Could you check a few things on this model? Use its own coordinates, in mm. Give positions to 0.01 mm unless a question says otherwise; leave off trailing zeros. Write each loop counter-clockwise with the first axis right and the second up, starting at its lowest first coordinate (ties: lowest second). Pieces come first, ordered by that corner, then holes. Notation, with made-up numbers: (-30.5, 7.25) - (17.5, 7.25) arc R36 ccw to (17.5, 45.25) - close; hole circle Ø5 at (39, 48). An arc over 180 degrees is marked (long way). Answer in a Markdown table with one row per item.
from build123d import *

# Parameters (mm, degrees)
F0_W     = 19
F0_H     = 35
F1_DEPTH = 6
F2_R     = 4
F3_R     = 3


with BuildPart() as f1:
    # F0 (on Front) → F1 (new body)
    with BuildSketch(Plane.XZ):
        with Locations((-4.541362, 17.316902)):
            Rectangle(F0_W, F0_H)
    extrude(amount=F1_DEPTH)

    # F2
    f2_edges = [f1.edges().sort_by_distance(p)[0] for p in [
        (4.958638, -3, 34.816902),
        (4.958638, -3, -0.183098),
        (-14.041362, -3, 34.816902),
        (-14.041362, -3, -0.183098),
    ]]
    fillet(f2_edges, radius=F2_R)

    # F3
    f3_edges = [f1.edges().sort_by_distance(p)[0] for p in [
        (-14.041362, -6, 17.316902),
    ]]
    fillet(f3_edges, radius=F3_R)


solid = f1.part
1) Imagine slicing it at B-B (x = -6.25). List the corners of the cut face in (y, z) for me.
Check values:
| item | result |
|---|---|
| outline | (-6, 2.82) arc R3 ccw to (-3, -0.18) - (0, -0.18) - (0, 34.82) - (-3, 34.82) arc R3 ccw to (-6, 31.82) - close |
2) Will these pins go through, and if not, where does the flat tip stop? P1, Ø2, axis at x = -9, y = -5, coming from the -Z side; P2, Ø5, axis at x = -10.5, z = 6, coming from the +Y side.
Check values:
| item | result |
|---|---|
| P1 | stops at z = -0.01 |
| P2 | stops at y = 0 |
3) Imagine slicing it at C-C (z = 26). List the corners of the cut face in (x, y) for me.
Check values:
| item | result |
|---|---|
| outline | (-14.04, -3) arc R3 ccw to (-11.04, -6) - (1.96, -6) arc R3 ccw to (4.96, -3) - (4.96, 0) - (-14.04, 0) - close |
4) Imagine slicing it at A-A (y = -1.6). List the corners of the cut face in (x, z) for me, then the cut area to 3 significant figures.
Check values:
| item | result |
|---|---|
| outline | (-14.04, 3.82) arc R4 ccw to (-10.04, -0.18) - (0.96, -0.18) arc R4 ccw to (4.96, 3.82) - (4.96, 30.82) arc R4 ccw to (0.96, 34.82) - (-10.04, 34.82) arc R4 ccw to (-14.04, 30.82) - close |
| area | 651 mm2 |
5) If I drill on line 1 (Z direction, x = 1, y = -3.85); line 2 (X direction, y = -4.5, z = 17); line 3 (X direction, y = -5.05, z = 22), over which ranges is the centre line in solid material (lowest first)?
Check values:
| item | result |
|---|---|
| line 1 | z = -0.06 to 34.69 |
| line 2 | x = -13.64 to 4.56 |
| line 3 | x = -13.23 to 4.15 |
